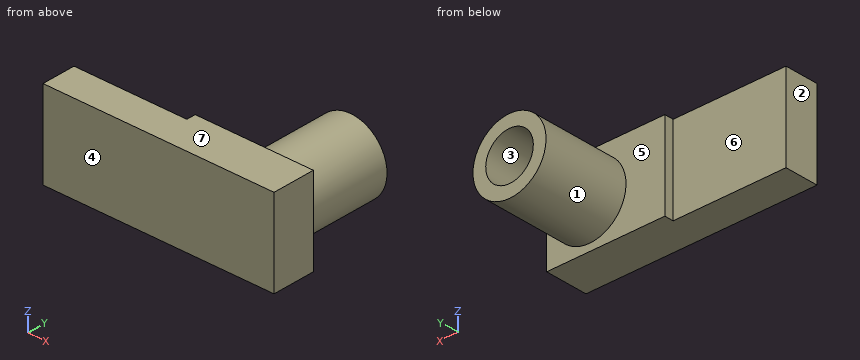
```python
from build123d import *

# Parameters (mm, degrees)
P_IDAT_VYSUNUT_M1_DEPTH = 30
SKICA2_R                = 25.104353528
SKICA2_R_2              = 16.352413197
P_IDAT_VYSUNUT_M2_DEPTH = 60


with BuildPart() as part:
    # Skica1 → Přidat vysunutím1 (new body, symmetric)
    with BuildSketch(Plane.XY):
        Polygon((0, 0), (0, 23.242356394), (77.561836829, 23.242356394), (77.561836829, 29.488625529), (158.739934736, 29.488625529), (158.739934736, 0), align=None)
    extrude(amount=P_IDAT_VYSUNUT_M1_DEPTH, both=True)

    # Skica2 → Přidat vysunutím2 (add)
    with BuildSketch(Plane(origin=(0, 29.488625529, 0), x_dir=(1, 0, 0), z_dir=(0, 1, 0))):
        with Locations(Location((129.340120448, 0, 0), (0, 0, 90))):  # turned: the seam where the file's is
            Circle(SKICA2_R)
        with Locations(Location((129.340120448, 0, 0), (0, 0, 270))):  # turned: the seam where the file's is
            Circle(SKICA2_R_2, mode=Mode.SUBTRACT)
    extrude(amount=P_IDAT_VYSUNUT_M2_DEPTH)


solid = part.part
```
Input: part model. Units: mm. Frame: model coordinates. Face numbers are marked on the shaded views. A direction names the side the tool comes from. Round coordinates to 2 decimals unless told otherwise and drop trailing zeros. Loops run counter-clockwise (first coordinate to the right, second up) from the corner with the lowest first, then second, coordinate; pieces in that order, holes last. Notation, with made-up numbers: (62.5, 1) -> (105.5, 1) arc R23 cw to (105.5, 12) -> close; hole circle Ø6 at (-26, 28). An arc over 180 degrees is marked (long way). Use one line per item in the form item = value. Start each with the question number.
Item 1: Contact query for flat-ended pins moving along their axis: pin 1 Ø12 at (y, z) = (28, 3.5) entering from -X; pin 2 Ø1.9 at (y, z) = (25.5, -5) entering from -X; pin 3 Ø6 at (y, z) = (51.5, 9) entering from +X; pin 4 Ø3 at (y, z) = (64.5, -18.5) entering from +X. Output: stop coordinate, or through.
Item 2: Section query B-B on x = 137.5. Return the cut outline in (y, z).
Item 3: Set-up query: the marked faces 5, 6 and 7. Return all of +Z, -Z, +X, -X, +Y, -Y with unobstructed straight access to the full face (end or side cutting, diameter ignored); none if empty.
Item 4: Section query C-C on y = 27.5. Return the cut outline in (x, z), then the cut area to 3 significant figures.
Item 5: Material intervals for L1, parallel to X at y = 75, z = 0; L2, parallel to Y at x = 101.5, z = 22; L3, parallel to X at y = 76, z = -14.5, sorted ascending. Write a range as from..to.
Item 6: Section query A-A on z = 0. Return the cut outline in (x, y), then the cut area to 3 significant figures.
Item 7: Mould query, pull axis X, two halves, no side actions, for the marked faces 1, 2, 3 and 4. Classes: pulls with the +X half, pulls with the -X half, needs draft (parallel to the pull), parting line crosses it, or undercut.
Item 8: Section query D-D on z = 19. Return the cut outline in (x, y), then the cut area to 3 significant figures.
Ans:
q1.pin_1 = 0
q1.pin_2 = 77.56
q1.pin_3 = 153.72
q1.pin_4 = 147.81
q2.outline = (0, -30) -> (29.49, -30) -> (29.49, -23.74) -> (89.49, -23.74) -> (89.49, -14.17) -> (29.49, -14.17) -> (29.49, 14.17) -> (89.49, 14.17) -> (89.49, 23.74) -> (29.49, 23.74) -> (29.49, 30) -> (0, 30) -> close
q3.face_5 = +Y
q3.face_6 = +Z, -Z, -X, +Y
q3.face_7 = +Z, +X, -X, +Y, -Y
q4.outline = (77.56, -30) -> (158.74, -30) -> (158.74, 30) -> (77.56, 30) -> close
q4.area = 4,870 mm^2
q5.L1 = 104.24..112.99, 145.69..154.44
q5.L2 = 0..29.49
q5.L3 = 108.85..121.78, 136.9..149.83
q6.outline = (0, 0) -> (158.74, 0) -> (158.74, 29.49) -> (154.44, 29.49) -> (154.44, 89.49) -> (145.69, 89.49) -> (145.69, 29.49) -> (112.99, 29.49) -> (112.99, 89.49) -> (104.24, 89.49) -> (104.24, 29.49) -> (77.56, 29.49) -> (77.56, 23.24) -> (0, 23.24) -> close
q6.area = 5,250 mm^2
q7.face_1 = parting line crosses it
q7.face_2 = pulls with the -X half
q7.face_3 = undercut
q7.face_4 = needs draft
q8.outline = (0, 0) -> (158.74, 0) -> (158.74, 29.49) -> (145.75, 29.49) -> (145.75, 89.49) -> (112.93, 89.49) -> (112.93, 29.49) -> (77.56, 29.49) -> (77.56, 23.24) -> (0, 23.24) -> close
q8.area = 6,170 mm^2
